from build123d import *

# Parameters (mm, degrees)
SKETCH1_W           = 200
SKETCH1_H           = 42
BOSS_EXTRUDE1_DEPTH = 6.35
SKETCH3_R           = 2
CUT_EXTRUDE2_DEPTH  = 7.35
SKETCH4_R           = 3.175
CUT_EXTRUDE3_DEPTH  = 7.35
CHAMFER1_SIZE       = 5
SKETCH9_R           = 3.175
CUT_EXTRUDE8_DEPTH  = 7.35
SKETCH10_R          = 12.5
CUT_EXTRUDE9_DEPTH  = 7.35
SKETCH12_R          = 3.302
CUT_EXTRUDE11_DEPTH = 7.35
SKETCH13_R          = 12.5
CUT_EXTRUDE12_DEPTH = 10


with BuildPart() as part:
    # Sketch1 → Boss-Extrude1 (new body)
    with BuildSketch(Plane.XY):
        Rectangle(SKETCH1_W, SKETCH1_H)
    extrude(amount=BOSS_EXTRUDE1_DEPTH)

    # Sketch3 → Cut-Extrude2 (cut, through all)
    with BuildSketch(Plane.XY.offset(6.35)):
        with Locations((-50, 10)):
            Circle(SKETCH3_R)
        with Locations((-50, -10)):
            Circle(SKETCH3_R)
    extrude(amount=-CUT_EXTRUDE2_DEPTH, mode=Mode.SUBTRACT)

    # Sketch4 → Cut-Extrude3 (cut, through all)
    with BuildSketch(Plane.XY.offset(6.35)):
        with Locations((-76, 0)):
            Circle(SKETCH4_R)
    extrude(amount=-CUT_EXTRUDE3_DEPTH, mode=Mode.SUBTRACT)

    # Chamfer1
    chamfer1_edges = [part.edges().sort_by_distance(p)[0] for p in [
        (100, -21, 3.175),
        (-100, -21, 3.175),
        (-100, 21, 3.175),
        (100, 21, 3.175),
    ]]
    chamfer(chamfer1_edges, length=CHAMFER1_SIZE)

    # Sketch9 → Cut-Extrude8 (cut, through all)
    with BuildSketch(Plane.XY.offset(6.35)):
        with Locations((80, 0)):
            Circle(SKETCH9_R)
    extrude(amount=-CUT_EXTRUDE8_DEPTH, mode=Mode.SUBTRACT)

    # Sketch10 → Cut-Extrude9 (cut, through all)
    with BuildSketch(Plane.XY.offset(6.35)):
        with Locations((80, 0)):
            Circle(SKETCH10_R)
    extrude(amount=-CUT_EXTRUDE9_DEPTH, mode=Mode.SUBTRACT)

    # Sketch12 → Cut-Extrude11 (cut, through all)
    with BuildSketch(Plane.XY.offset(6.35)):
        with Locations((-93, 0)):
            Circle(SKETCH12_R)
    extrude(amount=-CUT_EXTRUDE11_DEPTH, mode=Mode.SUBTRACT)

    # Sketch13 → Cut-Extrude12 (cut)
    with BuildSketch(Plane.XY.offset(6.35)):
        Polygon((45, 21), (50, 16), (50, -16), (45, -21), (95, -21), (100, -16), (100, 16), (95, 21), align=None)
        with Locations((80, 0)):
            Circle(SKETCH13_R, mode=Mode.SUBTRACT)
        with BuildLine():
            Line((-25, 7.46), (35, 7.46))
            ThreePointArc((35, 7.46), (37.54, 10), (35, 12.54))
            Line((35, 12.54), (-25, 12.54))
            ThreePointArc((-25, 12.54), (-27.54, 10), (-25, 7.46))
        make_face()
        with BuildLine():
            ThreePointArc((35, -7.46), (37.54, -10), (35, -12.54))
            Line((35, -12.54), (-25, -12.54))
            ThreePointArc((-25, -12.54), (-27.54, -10), (-25, -7.46))
            Line((-25, -7.46), (35, -7.46))
        make_face()
    extrude(amount=-CUT_EXTRUDE12_DEPTH, mode=Mode.SUBTRACT)


solid = part.part
The listing builds one solid part. Answer for the finished solid, in the listing's coordinates (mm). A direction names the side the tool comes from. Round coordinates to 2 decimals unless told otherwise and drop trailing zeros. Write each loop counter-clockwise with the first axis right and the second up, starting at its lowest first coordinate (ties: lowest second). Pieces come first, ordered by that corner, then holes. Notation, with made-up numbers: M -27.75,12 L 5.25,12 A21 cw 5.25,50 Z; hole C 15.25,-1 d9. An arc over 180 degrees is marked long. Write each question's results on one line, items separated by ' | '. Start each with the question number.
Item 1: Find section D-D on x = -76. Write down the section's boundary in (y, z) (3 decimals), and give its area (3 significant figures).
Item 2: Find section C-C on z = 5. Write down the section's boundary in (x, y) (3 decimals), and give its area (3 significant figures).
Item 3: Straight lines are drawn through the part: probe 1 along Y at (x, z) = (0.5, 5); probe 2 along Y at (x, z) = (-50, 5.25); probe 3 along Y at (x, z) = (-76, 1.5) (3 decimals). For each, find the intervals that lie inside material, in ascending order.
Item 4: Which of the six approach directions +Z, -Z, +X, -X, +Y, -Y give full straight-line access (tool end or side, diameter ignored) to faces 5 (the cylindrical face through (37.54, -9.94, 3.22)), 6 (the flat face through (-26, 0, 0))?
Item 5: Find section A-A on y = 0. Write down the section's boundary in (x, z) (3 decimals).
Item 6: Find section B-B on x = -50. Write down the section's boundary in (y, z), and give its area (3 significant figures).
Item 7: The mould has two halves that part along Y. Classify faces 1 (the cylindrical face through (37.54, 9.94, 3.22)), 2 (the flat face through (-100, 0, 3)), 3 (the cylindrical face through (-51.474, 11.352, 3.219)), 4 (the flat face through (-97, 19, 3)): +Y half, -Y half, draft (parallel to the pull), parting line (faces both ways), or undercut.
Item 8: Given pin 1 Ø6.5 at (x, y) = (-50, 10) entering from +Z, flat-ended and moving along its own axis, determine where the tip first touches the part or whether it passes through.
Answer block:
1) outline: M -21,0 L -3.175,0 L -3.175,6.35 L -21,6.35 Z; M 3.175,0 L 21,0 L 21,6.35 L 3.175,6.35 Z | area: 226 mm²
2) outline: M -100,-16 L -95,-21 L 45,-21 L 50,-16 L 50,16 L 45,21 L -95,21 L -100,16 Z; hole C -93,0 d6.604; hole C -76,0 d6.35; hole C -50,-10 d4; hole C -50,10 d4; hole M -25,-12.54 L 35,-12.54 A2.54 ccw 35,-7.46 L -25,-7.46 A2.54 ccw Z; hole M -25,7.46 L 35,7.46 A2.54 ccw 35,12.54 L -25,12.54 A2.54 ccw Z | area: 5,510 mm²
3) probe 1: y = -21 to -12.54, -7.46 to 7.46, 12.54 to 21 | probe 2: y = -21 to -12, -8 to 8, 12 to 21 | probe 3: y = -21 to -3.175, 3.175 to 21
4) face 5: +Z, -Z | face 6: -Z, +X, -X, +Y, -Y
5) outline: M -100,0 L -96.302,0 L -96.302,6.35 L -100,6.35 Z; M -89.698,0 L -79.175,0 L -79.175,6.35 L -89.698,6.35 Z; M -72.825,0 L 50,0 L 50,6.35 L -72.825,6.35 Z
6) outline: M -21,0 L -12,0 L -12,6.35 L -21,6.35 Z; M -8,0 L 8,0 L 8,6.35 L -8,6.35 Z; M 12,0 L 21,0 L 21,6.35 L 12,6.35 Z | area: 216 mm²
7) face 1: undercut | face 2: draft | face 3: undercut | face 4: +Y half
8) pin 1: stops at z = 6.35
